Read the model definition and answer for the solid it produces. Units are mm, in the model's axes. Face numbers are marked on the shaded views. A direction names the side the tool comes from. Coordinates: 2 decimals unless noted, no trailing zeros. Loops run counter-clockwise (first coordinate to the right, second up) from the corner with the lowest first, then second, coordinate; pieces in that order, holes last. Notation, with made-up numbers: M -18,3.25 L 30,3.25 A27 cw 30,29.25 Z; hole C 34.25,83.25 d7. An arc over 180 degrees is marked long. One line per item, written item: value. Start each with the question number.
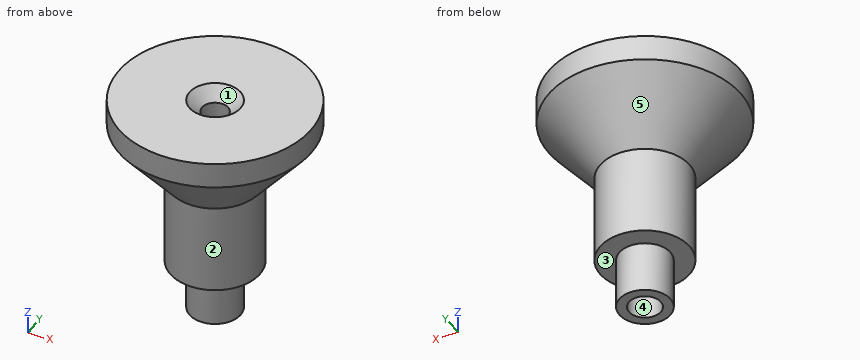
```python
from build123d import *

# Parameters (mm, degrees)
BROCA_DE_ROSQUEAR_PARA_TARRAXA_DE_M2_5X0_D = 2.05
FURO_ROSCADO_DE_M3X0_53_D                  = 2.5
FURO_ROSCADO_DE_M3X0_53_DEPTH              = 10
FURO_ROSCADO_DE_M3X0_53_TIP                = 0.751075774


with BuildPart() as part:
    # Esboço1 → Revolução1 (revolve)
    with BuildSketch(Plane(origin=(0, 0, 0), x_dir=(1, 0, 0), z_dir=(0, 1, 0))):
        Polygon((0, 0), (7.5, 0), (7.5, 2), (3.5, 6.75), (3.5, 13.75), (2, 13.75), (2, 17.75), (0, 17.75), align=None)
    revolve(axis=Axis((0, 0, 0), (0, 0, -1)))

    # Esboço8 → Corte-Revolução3 (revolve, cut)
    with BuildSketch(Plane(origin=(0, 0, 0), x_dir=(1, 0, 0), z_dir=(0, 1, 0))):
        Polygon((0, 0), (2, 0), (0, 2), align=None)
    revolve(axis=Axis((0, 0, -3.199109989), (0, 0, 1)), mode=Mode.SUBTRACT)

    # Broca de rosquear para tarraxa de M2.5x0.451 (through all)
    with Locations(Plane.XY):
        with Locations((0, 0)):
            Hole(BROCA_DE_ROSQUEAR_PARA_TARRAXA_DE_M2_5X0_D / 2)

    # Furo roscado de M3x0.53
    with Locations(Plane(origin=(0, 0, -17.75), x_dir=(-1, 0, 0), z_dir=(0, 0, -1))):
        with Locations((0, 0)):
            Hole(FURO_ROSCADO_DE_M3X0_53_D / 2, depth=FURO_ROSCADO_DE_M3X0_53_DEPTH)
            with Locations((0, 0, -(FURO_ROSCADO_DE_M3X0_53_DEPTH + FURO_ROSCADO_DE_M3X0_53_TIP / 2))):  # 118° drill point
                Cone(0, FURO_ROSCADO_DE_M3X0_53_D / 2, FURO_ROSCADO_DE_M3X0_53_TIP, mode=Mode.SUBTRACT)


solid = part.part
```
1) A tool of negligible diameter and unlimited length cuts with its end or side. For the marked faces 1 and 2, from which of +Z, -Z, +X, -X, +Y, -Y can it reach the whole face along a straight path? Write none if from no direction.
2) For a pull along Y with two mould halves and no side action, classify the marked faces 3, 4 and 5 as released by +Y, released by -Y, zero draft, split by the parting line, or undercut.
3) Section A-A (y = 0) is taken. Determine the outline of the cut face in (x, z) (3 decimals).
4) Consider line 1 along Y through (x, z) = (0, -12.5); line 2 along Y through (x, z) = (0, -15.25). Determine where each line is inside the solid, lowest interval first.
5) Section C-C (z = -7.25) is taken. Determine the outline of the cut face in (x, y) (3 decimals).
6) Flat-ended cylindrical pins translate along their axes: pin 1 (2 mm diameter, centred on y = 2, z = -11, fed in from +X); pin 2 (5 mm diameter, centred on y = 0.5, z = -7.5, fed in from -X); pin 3 (5 mm diameter, centred on y = 4.5, z = -4, fed in from -X); pin 4 (1.6 mm diameter, centred on x = 0, y = 0, fed in from -Z). Find the tip coordinate at first contact, or state that the pin passes through.
7) Section D-D (z = -13.5) is taken. Determine the outline of the cut face in (x, y), then the cut area to 3 significant figures.
Results found:
1. face 1: +Z
1. face 2: -Z
2. face 3: zero draft
2. face 4: undercut
2. face 5: split by the parting line
3. outline: M -7.5,-2 L -3.5,-6.75 L -3.5,-13.75 L -2,-13.75 L -2,-17.75 L -1.25,-17.75 L -1.25,-7.75 L -1.025,-7.615 L -1.025,-0.975 L -2,0 L -7.5,0 Z; M 1.025,-7.615 L 1.25,-7.75 L 1.25,-17.75 L 2,-17.75 L 2,-13.75 L 3.5,-13.75 L 3.5,-6.75 L 7.5,-2 L 7.5,0 L 2,0 L 1.025,-0.975 Z
4. line 1: y = -3.5 to -1.25, 1.25 to 3.5
4. line 2: y = -2 to -1.25, 1.25 to 2
5. outline: C 0,0 d7; hole C 0,0 d2.05
6. pin 1: stops at x = 3.35
6. pin 2: stops at x = -4.96
6. pin 3: stops at x = -6.87
6. pin 4: passes through
7. outline: C 0,0 d7; hole C 0,0 d2.5
7. area: 33.6 mm²
